Read the model definition and answer for the solid it produces. Units are mm, in the model's axes. Face numbers are marked on the shaded views. A direction names the side the tool comes from. Coordinates: 2 decimals unless noted, no trailing zeros. Loops run counter-clockwise (first coordinate to the right, second up) from the corner with the lowest first, then second, coordinate; pieces in that order, holes last. Notation, with made-up numbers: (63, -35.5) -> (81, -35.5) arc R21 ccw to (81, -29.5) -> close; hole circle Ø11 at (71.5, -5). An arc over 180 degrees is marked (long way). Answer as a JSON object with one key per item and string values. Group by question number.
Q1. The part is cut by section A-A on y = 1.25. Write down the section's boundary in (x, z).
Q2. The part is cut by section C-C on z = 2.25. Write down the section's boundary in (x, y), and give its area (3 significant figures).
Q3. The part is cut by section B-B on x = -1. Write down the section's boundary in (y, z).
Q4. Each of these flat-tipped pins is pushed along its axis until it touches: P1, Ø2, axis at y = 1, z = 0, coming from the -X side; P2, Ø1.2, axis at y = 1.5, z = 0, coming from the +X side; P3, Ø1.5, axis at y = 2.5, z = 4.5, coming from the +X side; P4, Ø1.2, axis at x = 0.5, z = -1, coming from the -Y side. Where does it stop, or does it pass through?
Q5. Determine the mould class of the marked faces 3, 4, 5 and 6 for opening direction X: released by +X, released by -X, zero draft, split by the parting line, or undercut.
Q6. Straight lines are drawn through the part: line 1 along Y through (x, z) = (7, 5.25); line 2 along Z through (x, y) = (-2.25, 2). For each, find the intervals that lie inside material, in ascending order. Write a range as [from, to].
Q7. The part is cut by section D-D on x = -4.5. Write down the section's boundary in (y, z).
Q8. For the marked faces 1 and 2, determine the directions among +Z, -Z, +X, -X, +Y, -Y from which every point of the face is accessible in a straight line to the end or side of a thin tool.
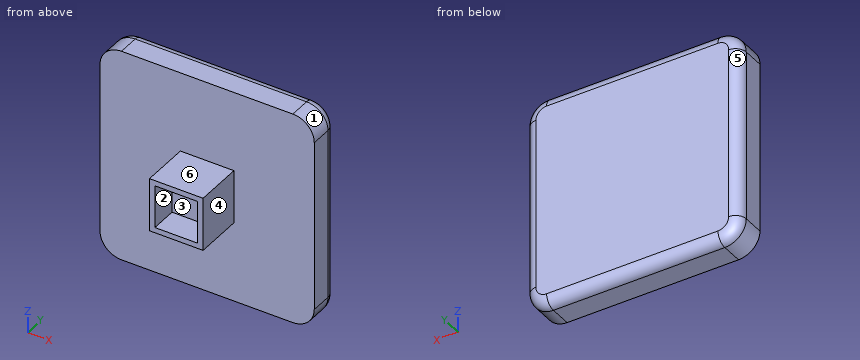
from build123d import *

# Parameters (mm, degrees)
SKETCH_1_W          = 5
SKETCH_1_H          = 5
EXTRUDE_1_DEPTH     = 2.5
SKETCH_2_W          = 4
SKETCH_2_H          = 4
CUT_EXTRUDE_1_DEPTH = 2.5
SKETCH_4_W          = 5
SKETCH_4_H          = 5
EXTRUDE_3_DEPTH     = 2
SKETCH_5_W          = 20
SKETCH_5_H          = 20
EXTRUDE_4_DEPTH     = 3
FILLET_6_R          = 2
FILLET_7_R          = 1


with BuildPart() as part:
    # 스케치1 → 보스-돌출1 (new body)
    with BuildSketch(Plane(origin=(0, 0, 0), x_dir=(1, 0, 0), z_dir=(0, 1, 0))):
        Rectangle(SKETCH_1_W, SKETCH_1_H)
    extrude(amount=EXTRUDE_1_DEPTH)

    # 스케치2 → 컷-돌출1 (cut)
    with BuildSketch(Plane(origin=(0, 2.5, 0), x_dir=(1, 0, 0), z_dir=(0, 1, 0))):
        Rectangle(SKETCH_2_W, SKETCH_2_H)
    extrude(amount=-CUT_EXTRUDE_1_DEPTH, mode=Mode.SUBTRACT)

    # 스케치4 → 보스-돌출3 (add)
    with BuildSketch(Plane(origin=(0, 2.5, 0), x_dir=(1, 0, 0), z_dir=(0, 1, 0))):
        Rectangle(SKETCH_4_W, SKETCH_4_H)
    extrude(amount=EXTRUDE_3_DEPTH)

    # 스케치5 → 보스-돌출4 (add)
    with BuildSketch(Plane(origin=(0, 4.5, 0), x_dir=(1, 0, 0), z_dir=(0, 1, 0))):
        Rectangle(SKETCH_5_W, SKETCH_5_H)
    extrude(amount=EXTRUDE_4_DEPTH)

    # 필렛6
    fillet_6_edges = [part.edges().sort_by_distance(p)[0] for p in [
        (10, 6, 10),
        (10, 6, -10),
        (-10, 6, -10),
        (-10, 6, 10),
    ]]
    fillet(fillet_6_edges, radius=FILLET_6_R)

    # 필렛7
    fillet_7_edges = [part.edges().sort_by_distance(p)[0] for p in [
        (-10, 7.5, 0),
        (0, 7.5, -10),
        (10, 7.5, 0),
        (0, 7.5, 10),
        (-9.414213562, 7.5, 9.414213562),
        (9.414213562, 7.5, 9.414213562),
        (9.414213562, 7.5, -9.414213562),
        (-9.414213562, 7.5, -9.414213562),
    ]]
    fillet(fillet_7_edges, radius=FILLET_7_R)


solid = part.part
Final values:
{
 "1": {"outline": "(-2.5, -2.5) -> (2.5, -2.5) -> (2.5, 2.5) -> (-2.5, 2.5) -> close; hole (-2, -2) -> (2, -2) -> (2, 2) -> (-2, 2) -> close"},
 "2": {"outline": "(-10, 4.5) -> (-2.5, 4.5) -> (-2.5, 0) -> (2.5, 0) -> (2.5, 4.5) -> (10, 4.5) -> (10, 6.5) arc R1 ccw to (9, 7.5) -> (-9, 7.5) arc R1 ccw to (-10, 6.5) -> close", "area": "82.1 mm2"},
 "3": {"outline": "(0, -2.5) -> (4.5, -2.5) -> (4.5, -10) -> (6.5, -10) arc R1 ccw to (7.5, -9) -> (7.5, 9) arc R1 ccw to (6.5, 10) -> (4.5, 10) -> (4.5, 2.5) -> (0, 2.5) -> (0, 2) -> (2.5, 2) -> (2.5, -2) -> (0, -2) -> close"},
 "4": {"P1": "stops at x = -2.5", "P2": "stops at x = 2.5", "P3": "passes through", "P4": "stops at y = 2.5"},
 "5": {"face 3": "undercut", "face 4": "released by +X", "face 5": "released by -X", "face 6": "zero draft"},
 "6": {"line 1": "y = [4.5, 7.5]", "line 2": "z = [-2.5, 2.5]"},
 "7": {"outline": "(4.5, -10) -> (6.5, -10) arc R1 ccw to (7.5, -9) -> (7.5, 9) arc R1 ccw to (6.5, 10) -> (4.5, 10) -> close"},
 "8": {"face 1": "+Z, +X, +Y, -Y", "face 2": "-Y"}
}
